Work out the finished part from the listing and answer in its coordinate system (mm). Face numbers are marked on the shaded views. A direction names the side the tool comes from. Round coordinates to 2 decimals unless told otherwise and drop trailing zeros. Loops run counter-clockwise (first coordinate to the right, second up) from the corner with the lowest first, then second, coordinate; pieces in that order, holes last. Notation, with made-up numbers: (70, -27.75) -> (117, -27.75) arc R27 ccw to (117, 4.25) -> close; hole circle Ø6 at (9, 48). An arc over 180 degrees is marked (long way). Use CSV: the item, a comma, the result in double quotes. Start each with the question number.
from build123d import *

# Parameters (mm, degrees)
SKETCH1_W            = 160.5788
SKETCH1_H            = 37.338
BOSS_EXTRUDE1_DEPTH  = 27.94
SKETCH2_W            = 157.5308
SKETCH2_H            = 34.29
CUT_EXTRUDE3_DEPTH   = 26.289
FILLET1_R            = 2.54
FILLET2_R            = 1.27
SKETCH3_W            = 46.228
SKETCH3_H            = 27.94
BOSS_EXTRUDE2_DEPTH  = 27.686
SKETCH8_W            = 44.704
SKETCH8_H            = 24.892
CUT_EXTRUDE6_DEPTH   = 27.686
CUT_EXTRUDE5_REACH   = 93.501
SKETCH7_R            = 9.525
CUT_EXTRUDE7_REACH   = 121.521
SKETCH9_W            = 23.876
SKETCH9_H            = 15.24
SKETCH10_R           = 2.54
SKETCH10_W           = 1.524
SKETCH10_H           = 3.556
BOSS_EXTRUDE5_DEPTH  = 7.62
SKETCH11_R           = 1.4605
BOSS_EXTRUDE6_DEPTH  = 1.651
CUT_EXTRUDE8_REACH   = 95.28
SKETCH12_W           = 8.218436834
SKETCH12_H           = 3.333271446
SKETCH13_R           = 1.524
BOSS_EXTRUDE7_DEPTH  = 26.162
SKETCH14_R           = 1.27
BOSS_EXTRUDE8_DEPTH  = 2.54
SKETCH15_W           = 1.524
SKETCH15_H           = 5.08
BOSS_EXTRUDE9_DEPTH  = 12.446
SKETCH16_OUTSIDE_W   = 196.104
SKETCH16_OUTSIDE_H   = 72.864
SKETCH16_OUTSIDE_W_2 = 159.0548
SKETCH16_OUTSIDE_H_2 = 35.814
CUT_EXTRUDE9_DEPTH   = 1.778
FILLET3_R            = 1.524
SKETCH17_W           = 5.334
SKETCH17_H           = 0.762
CUT_EXTRUDE10_DEPTH  = 8.89
SKETCH18_W           = 4.064
SKETCH18_H           = 3.81
CUT_EXTRUDE11_DEPTH  = 1.016


with BuildPart() as part:
    # Sketch1 → Boss-Extrude1 (new body)
    with BuildSketch(Plane(origin=(0, 0, 0), x_dir=(1, 0, 0), z_dir=(0, 1, 0))):
        Rectangle(SKETCH1_W, SKETCH1_H)
    extrude(amount=BOSS_EXTRUDE1_DEPTH)

    # Sketch2 → Cut-Extrude3 (cut)
    with BuildSketch(Plane(origin=(0, 27.94, 0), x_dir=(1, 0, 0), z_dir=(0, 1, 0))):
        Rectangle(SKETCH2_W, SKETCH2_H)
    extrude(amount=-CUT_EXTRUDE3_DEPTH, mode=Mode.SUBTRACT)

    # Fillet1
    fillet1_edges = [part.edges().sort_by_distance(p)[0] for p in [
        (0, 0, 18.669),
        (-80.2894, 0, 0),
        (0, 0, -18.669),
        (80.2894, 0, 0),
        (80.2894, 13.97, 18.669),
        (-80.2894, 13.97, 18.669),
        (-80.2894, 13.97, -18.669),
        (80.2894, 13.97, -18.669),
    ]]
    fillet(fillet1_edges, radius=FILLET1_R)

    # Fillet2
    fillet2_edges = [part.edges().sort_by_distance(p)[0] for p in [
        (-78.7654, 14.7955, -17.145),
        (-78.7654, 14.7955, 17.145),
        (78.7654, 14.7955, 17.145),
        (78.7654, 14.7955, -17.145),
    ]]
    fillet(fillet2_edges, radius=FILLET2_R)

    # Sketch3 → Boss-Extrude2 (add)
    with BuildSketch(Plane(origin=(0, 1.651, 0), x_dir=(1, 0, 0), z_dir=(0, 1, 0))):
        with Locations((-55.6514, 0)):
            Rectangle(SKETCH3_W, SKETCH3_H)
    extrude(amount=BOSS_EXTRUDE2_DEPTH)

    # Sketch8 → Cut-Extrude6 (cut)
    with BuildSketch(Plane(origin=(0, 29.337, 0), x_dir=(1, 0, 0), z_dir=(0, 1, 0))):
        with Locations((-56.4134, 0)):
            Rectangle(SKETCH8_W, SKETCH8_H)
    extrude(amount=-CUT_EXTRUDE6_DEPTH, mode=Mode.SUBTRACT)

    # Cut-Extrude5: up to this face of the body (flat: up to its plane)
    cut_extrude5_end = Plane(part.part.faces().sort_by_distance((-55.6514, 15.494, -13.97))[0])
    # Sketch7 → Cut-Extrude5 (cut, up to the picked face)
    with BuildSketch(Plane.XY.offset(13.97), mode=Mode.PRIVATE) as cut_extrude5_sk1:
        with Locations((-55.6514, 29.337)):
            Circle(SKETCH7_R)
    cut_extrude5_tool1 = split(extrude(cut_extrude5_sk1.sketch, amount=-CUT_EXTRUDE5_REACH, mode=Mode.PRIVATE), bisect_by=cut_extrude5_end, keep=Keep.BOTH, mode=Mode.PRIVATE)
    add(cut_extrude5_tool1.solids().sort_by(Axis((-55.6514, 29.337, 13.97), (0, 0, -1)))[0], mode=Mode.SUBTRACT)

    # Sketch9 → Cut-Extrude7 (cut, up to next)
    with BuildSketch(Plane.ZY.offset(34.0614), mode=Mode.PRIVATE) as cut_extrude7_sk1:
        with Locations((0, 21.717)):
            Rectangle(SKETCH9_W, SKETCH9_H)
    cut_extrude7_tool1 = extrude(cut_extrude7_sk1.sketch, amount=-CUT_EXTRUDE7_REACH, mode=Mode.PRIVATE) & part.part
    add(cut_extrude7_tool1.solids().sort_by_distance((-34.0614, 21.717, 0))[0], mode=Mode.SUBTRACT)

    # Sketch10 → Boss-Extrude5 (add)
    with BuildSketch(Plane(origin=(0, 1.651, 0), x_dir=(1, 0, 0), z_dir=(0, 1, 0))):
        with Locations(Location((-19.5834, 0, 0), (0, 0, 90))):
            Circle(SKETCH10_R)
        with Locations(Location((17.5006, 0, 0), (0, 0, 90))):
            Circle(SKETCH10_R)
        with Locations((-14.5034, 15.367)):
            Rectangle(SKETCH10_W, SKETCH10_H)
        with Locations((12.4206, 15.367)):
            Rectangle(SKETCH10_W, SKETCH10_H)
        with Locations((-14.5034, -15.367)):
            Rectangle(SKETCH10_W, SKETCH10_H)
        with Locations((12.4206, -15.367)):
            Rectangle(SKETCH10_W, SKETCH10_H)
    extrude(amount=BOSS_EXTRUDE5_DEPTH)

    # Sketch11 → Boss-Extrude6 (add)
    with BuildSketch(Plane(origin=(0, 9.271, 0), x_dir=(1, 0, 0), z_dir=(0, 1, 0))):
        with Locations(Location((17.5006, 0, 0), (0, 0, 90))):
            Circle(SKETCH11_R)
        with Locations(Location((-19.5834, 0, 0), (0, 0, 90))):
            Circle(SKETCH11_R)
    extrude(amount=BOSS_EXTRUDE6_DEPTH)

    # Sketch12 → Cut-Extrude8 (cut, up to next)
    with BuildSketch(Plane.XY.offset(18.669), mode=Mode.PRIVATE) as cut_extrude8_sk1:
        with Locations((-19.030181583, 12.461635723)):
            Rectangle(SKETCH12_W, SKETCH12_H)
    cut_extrude8_tool1 = extrude(cut_extrude8_sk1.sketch, amount=-CUT_EXTRUDE8_REACH, mode=Mode.PRIVATE) & part.part
    add(cut_extrude8_tool1.solids().sort_by_distance((-19.030182, 12.461636, 18.669))[0], mode=Mode.SUBTRACT)

    # Sketch13 → Boss-Extrude7 (add)
    with BuildSketch(Plane(origin=(0, 1.651, 0), x_dir=(1, 0, 0), z_dir=(0, 1, 0))):
        with Locations(Location((32.7914, 10.033, 0), (0, 0, 90))):
            Circle(SKETCH13_R)
        with Locations(Location((75.9714, 10.033, 0), (0, 0, 90))):
            Circle(SKETCH13_R)
        with Locations(Location((75.9714, -10.033, 0), (0, 0, 90))):
            Circle(SKETCH13_R)
        with Locations(Location((32.7914, -10.033, 0), (0, 0, 90))):
            Circle(SKETCH13_R)
    extrude(amount=BOSS_EXTRUDE7_DEPTH)

    # Sketch14 → Boss-Extrude8 (add)
    with BuildSketch(Plane(origin=(0, 27.813, 0), x_dir=(1, 0, 0), z_dir=(0, 1, 0))):
        with Locations(Location((32.7914, 10.033, 0), (0, 0, 270))):
            Circle(SKETCH14_R)
        with Locations(Location((32.7914, -10.033, 0), (0, 0, 270))):
            Circle(SKETCH14_R)
        with Locations(Location((75.9714, -10.033, 0), (0, 0, 270))):
            Circle(SKETCH14_R)
        with Locations(Location((75.9714, 10.033, 0), (0, 0, 270))):
            Circle(SKETCH14_R)
    extrude(amount=BOSS_EXTRUDE8_DEPTH)

    # Sketch15 → Boss-Extrude9 (add)
    with BuildSketch(Plane(origin=(0, 1.651, 0), x_dir=(1, 0, 0), z_dir=(0, 1, 0))):
        with Locations((-43.7134, 9.906)):
            Rectangle(SKETCH15_W, SKETCH15_H)
        with Locations((-43.7134, -9.906)):
            Rectangle(SKETCH15_W, SKETCH15_H)
        with Locations((-69.1134, 9.906)):
            Rectangle(SKETCH15_W, SKETCH15_H)
        with Locations((-69.1134, -9.906)):
            Rectangle(SKETCH15_W, SKETCH15_H)
    extrude(amount=BOSS_EXTRUDE9_DEPTH)

    # Sketch16 outside → Cut-Extrude9 (cut)
    with BuildSketch(Plane(origin=(0, 27.94, 0), x_dir=(1, 0, 0), z_dir=(0, 1, 0))):
        Rectangle(SKETCH16_OUTSIDE_W, SKETCH16_OUTSIDE_H)
        Rectangle(SKETCH16_OUTSIDE_W_2, SKETCH16_OUTSIDE_H_2, mode=Mode.SUBTRACT)
    extrude(amount=-CUT_EXTRUDE9_DEPTH, mode=Mode.SUBTRACT)

    # Fillet3
    fillet3_edges = [part.edges().sort_by_distance(p)[0] for p in [
        (-79.5274, 27.051, -17.907),
        (79.5274, 27.051, -17.907),
        (79.5274, 27.051, 17.907),
        (-79.5274, 27.051, 17.907),
    ]]
    fillet(fillet3_edges, radius=FILLET3_R)

    # Sketch17 → Cut-Extrude10 (cut)
    with BuildSketch(Plane(origin=(0, 27.94, 0), x_dir=(1, 0, 0), z_dir=(0, 1, 0))):
        with Locations((74.8284, -17.526)):
            Rectangle(SKETCH17_W, SKETCH17_H)
    extrude(amount=-CUT_EXTRUDE10_DEPTH, mode=Mode.SUBTRACT)

    # Sketch18 → Cut-Extrude11 (cut)
    with BuildSketch(Plane(origin=(0, 0, 17.145), x_dir=(-1, 0, 0), z_dir=(0, 0, -1))):
        with Locations((-0.0254, 20.447)):
            Rectangle(SKETCH18_W, SKETCH18_H)
    cut_extrude11 = extrude(amount=-CUT_EXTRUDE11_DEPTH, mode=Mode.SUBTRACT)

    # Mirror1: Cut-Extrude11 across plane
    add(cut_extrude11.mirror(Plane.XY), mode=Mode.SUBTRACT)


solid = part.part
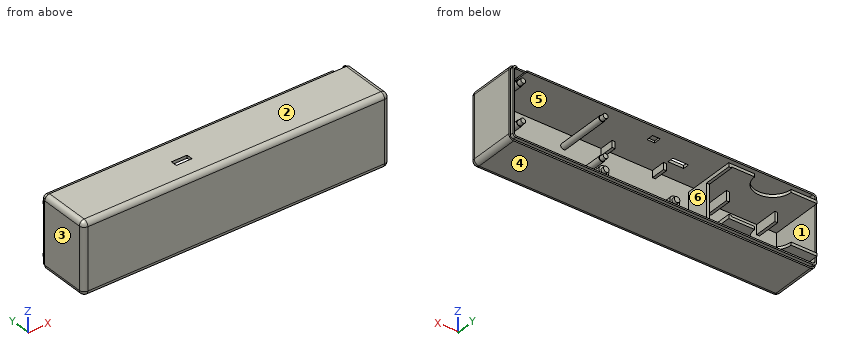
Q1. Section B-B, the plane x = 29 is taken. Write down the section's boundary in (y, z) (3 decimals), and give its area (3 significant figures).
Q2. Section C-C, the plane y = 6 is taken. Give the number of separate pieces and of enclosed holes in the cut face, and give its area (3 significant figures).
Q3. Which of the six approach directions +Z, -Z, +X, -X, +Y, -Y give full straight-line access (tool end or side, diameter ignored) to the marked faces 1 and 2?
Q4. Each of these flat-tipped pins is pushed along its axis until it touches: pin 1 (0.8 mm diameter, centred on x = -0.5, z = 18, fed in from +Y); pin 2 (1.2 mm diameter, centred on x = -14.5, z = 15, fed in from +Y); pin 3 (1.5 mm diameter, centred on x = 17, z = -0.5, fed in from +Y). Where does it stop, or does it pass through?
Q5. Straight lines are drawn through the part: line 1 (Z direction, x = -41.5, y = 3.5) (3 decimals); line 2 (X direction, y = 3, z = 7.5); line 3 (X direction, y = 26.5, z = 2.5). For each, find the intervals that lie inside material, in ascending order. Write a range as from..to.
Q6. For a pull along X with two mould halves and no side action, classify the marked faces 3, 4, 5 and 6 as pulls with the +X half, pulls with the -X half, needs draft (parallel to the pull), parting line crosses it, or undercut.
Q7. Section D-D, the plane x = -37.5 is taken. Write down the section's boundary in (y, z) (3 decimals), and give its area (3 significant figures).
Q8. Section A-A, the plane z = -5.5 is taken. Write down the section's boundary in (x, y), and give its area (3 significant figures).
Report:
1,outline,"(0, -16.129) arc R2.54 ccw to (2.54, -18.669) -> (26.162, -18.669) -> (26.162, -17.907) -> (27.94, -17.907) -> (27.94, -17.145) -> (1.651, -17.145) -> (1.651, 17.145) -> (27.94, 17.145) -> (27.94, 17.907) -> (26.162, 17.907) -> (26.162, 18.669) -> (2.54, 18.669) arc R2.54 ccw to (0, 16.129) -> close"
1,area,"136 mm²"
2,separate pieces,"7"
2,enclosed holes,"2"
2,area,"891 mm²"
3,face 1,"+Y"
3,face 2,"+Z, +X, -X, +Y, -Y"
4,pin 1,"stops at y = 27.94"
4,pin 2,"stops at y = 9.27"
4,pin 3,"stops at y = 10.92"
5,line 1,"z = -18.669..-17.145, -13.97..-12.446, 12.446..13.97, 17.145..18.669"
5,line 2,"x = -80.29..-78.77, -69.88..-68.35, -44.48..-42.95, -34.06..-32.54, 78.77..80.29"
5,line 3,"x = -79.53..-78.77, 78.77..79.53"
6,face 3,"pulls with the -X half"
6,face 4,"needs draft"
6,face 5,"undercut"
6,face 6,"undercut"
7,outline,"(0, -16.129) arc R2.54 ccw to (2.54, -18.669) -> (26.162, -18.669) -> (26.162, -17.907) -> (27.94, -17.907) -> (27.94, -17.145) -> (1.651, -17.145) -> (1.651, -13.97) -> (29.337, -13.97) -> (29.337, -12.446) -> (1.651, -12.446) -> (1.651, 12.446) -> (29.337, 12.446) -> (29.337, 13.97) -> (1.651, 13.97) -> (1.651, 17.145) -> (27.94, 17.145) -> (27.94, 17.907) -> (26.162, 17.907) -> (26.162, 18.669) -> (2.54, 18.669) arc R2.54 ccw to (0, 16.129) -> close"
7,area,"221 mm²"
8,outline,"(-80.29, 2.54) arc R2.54 ccw to (-77.75, 0) -> (77.75, 0) arc R2.54 ccw to (80.29, 2.54) -> (80.29, 26.16) -> (79.53, 26.16) -> (79.53, 27.94) -> (78.77, 27.94) -> (78.77, 1.65) -> (-32.54, 1.65) -> (-32.54, 14.1) -> (-34.06, 14.1) -> (-34.06, 1.65) -> (-78.77, 1.65) -> (-78.77, 27.94) -> (-79.53, 27.94) -> (-79.53, 26.16) -> (-80.29, 26.16) -> close"
8,area,"359 mm²"
